Check sheet for the modelled part. Datum: model origin and axes. Units: mm. Give positions to 0.01 mm unless a question says otherwise; leave off trailing zeros. Order: outer loops, then holes, each group sorted by start corner. A loop starts at its lowest first (then second) coordinate and runs counter-clockwise, first axis right, second up.
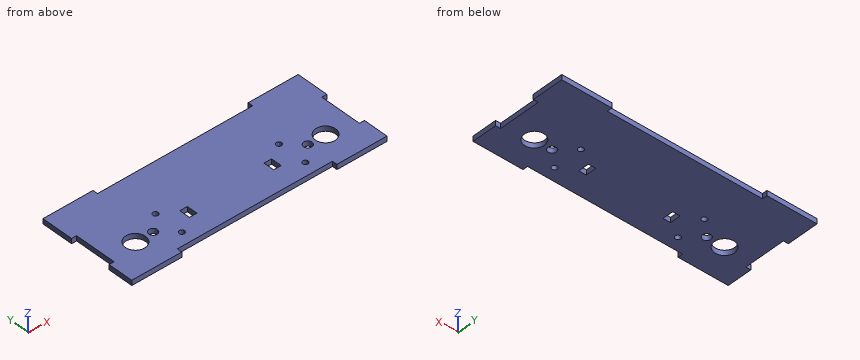
from build123d import *

# Parameters (mm, degrees)
ESBO_O1_W                = 153
ESBO_O1_H                = 59
RESSALTO_EXTRUS_O1_DEPTH = 3
ESBO_O2_W                = 93
ESBO_O2_H                = 3
CORTE_EXTRUS_O1_DEPTH    = 83.045718962
ESBO_O3_W                = 3
ESBO_O3_H                = 25
CORTE_EXTRUS_O2_DEPTH    = 83.045718962
ESBO_O4_R                = 6
CORTE_EXTRUS_O3_DEPTH    = 83.045718962
ESBO_O5_R                = 1.6
ESBO_O5_R_2              = 2.5
ESBO_O5_W                = 4.5
ESBO_O5_H                = 6.4
CORTE_EXTRUS_O4_DEPTH    = 83.045718962


with BuildPart() as part:
    # Esboço1 → Ressalto-extrusão1 (new body)
    with BuildSketch(Plane.XY):
        Rectangle(ESBO_O1_W, ESBO_O1_H)
    extrude(amount=RESSALTO_EXTRUS_O1_DEPTH)

    # Esboço2 → Corte-extrusão1 (cut, through all)
    with BuildSketch(Plane.XY.offset(3)):
        with Locations((0, 28)):
            Rectangle(ESBO_O2_W, ESBO_O2_H)
        with Locations((0, -28)):
            Rectangle(ESBO_O2_W, ESBO_O2_H)
    extrude(amount=-CORTE_EXTRUS_O1_DEPTH, mode=Mode.SUBTRACT)

    # Esboço3 → Corte-extrusão2 (cut, through all)
    with BuildSketch(Plane.XY.offset(3)):
        with Locations((-75, -2)):
            Rectangle(ESBO_O3_W, ESBO_O3_H)
        with Locations((75, -2)):
            Rectangle(ESBO_O3_W, ESBO_O3_H)
    extrude(amount=-CORTE_EXTRUS_O2_DEPTH, mode=Mode.SUBTRACT)

    # Esboço4 → Corte-extrusão3 (cut, through all)
    with BuildSketch(Plane(origin=(0, 0, 0), x_dir=(-1, 0, 0), z_dir=(0, 0, -1))):
        with Locations((57, -10.3)):
            Circle(ESBO_O4_R)
        with Locations(Location((-57, -10.3, 0), (0, 0, 180))):
            Circle(ESBO_O4_R)
    extrude(amount=-CORTE_EXTRUS_O3_DEPTH, mode=Mode.SUBTRACT)

    # Esboço5 → Corte-extrusão4 (cut, through all)
    with BuildSketch(Plane.XY):
        with Locations(Location((-37, -1.55, 0), (0, 0, 180))):
            Circle(ESBO_O5_R)
        with Locations(Location((-37, -19.05, 0), (0, 0, 180))):
            Circle(ESBO_O5_R)
        with Locations(Location((37, -19.05, 0), (0, 0, 180))):
            Circle(ESBO_O5_R)
        with Locations(Location((37, -1.55, 0), (0, 0, 180))):
            Circle(ESBO_O5_R)
        with Locations(Location((-46.35, -10.3, 0), (0, 0, 180))):
            Circle(ESBO_O5_R_2)
        with Locations(Location((46.35, -10.3, 0), (0, 0, 180))):
            Circle(ESBO_O5_R_2)
        with Locations((25.25, -10.3)):
            Rectangle(ESBO_O5_W, ESBO_O5_H)
        with Locations((-25.25, -10.3)):
            Rectangle(ESBO_O5_W, ESBO_O5_H)
    extrude(amount=CORTE_EXTRUS_O4_DEPTH, mode=Mode.SUBTRACT)


solid = part.part
1) Material ranges on L1, parallel to Y at x = -37, z = 1.7; L2, parallel to Y at x = 26.5, z = 2.65; L3, parallel to Y at x = 57, z = 2.1, recorded low to high.
Recorded:
L1: y = -26.5 to -20.65, -17.45 to -3.15, 0.05 to 26.5
L2: y = -26.5 to -13.5, -7.1 to 26.5
L3: y = -29.5 to -16.3, -4.3 to 29.5
2) Section check C-C, the plane y = -19.05. Record the cut outline in (x, z), then the cut area to 3 significant figures.
Recorded:
outline: (-76.5, 0) - (-38.6, 0) - (-38.6, 3) - (-76.5, 3) - close; (-35.4, 0) - (35.4, 0) - (35.4, 3) - (-35.4, 3) - close; (38.6, 0) - (76.5, 0) - (76.5, 3) - (38.6, 3) - close
area: 440 mm2
3) Section check B-B, the plane y = -10.3. Record the cut outline in (x, z).
Recorded:
outline: (-73.5, 0) - (-63, 0) - (-63, 3) - (-73.5, 3) - close; (-51, 0) - (-48.85, 0) - (-48.85, 3) - (-51, 3) - close; (-43.85, 0) - (-27.5, 0) - (-27.5, 3) - (-43.85, 3) - close; (-23, 0) - (23, 0) - (23, 3) - (-23, 3) - close; (27.5, 0) - (43.85, 0) - (43.85, 3) - (27.5, 3) - close; (48.85, 0) - (51, 0) - (51, 3) - (48.85, 3) - close; (63, 0) - (73.5, 0) - (73.5, 3) - (63, 3) - close
4) Section check D-D, the plane z = 0.8. State how many separate pieces and enclosed holes the cut face has, then the cut area to 3 significant figures.
Recorded:
separate pieces: 1
enclosed holes: 10
area: 7,960 mm2
5) Depth check by flat-ended pin: pin 1 Ø1 at (y, z) = (-0.5, 1.5) entering from -X; pin 2 Ø0.9 at (x, z) = (-24.5, 2) entering from -Y. Enter the tip coordinate at first touch or a pass-through.
Recorded:
pin 1: stops at x = -73.5
pin 2: stops at y = -26.5
6) Section check A-A, the plane x = -57. Record the cut outline in (y, z).
Recorded:
outline: (-29.5, 0) - (-16.3, 0) - (-16.3, 3) - (-29.5, 3) - close; (-4.3, 0) - (29.5, 0) - (29.5, 3) - (-4.3, 3) - close
